```python
from build123d import *

# Parameters (mm, degrees)
F0_R     = 100
F1_DEPTH = 25
F3_DEPTH = 25.5
F4_SIZE  = 5
F5_R     = 5
F6_R     = 30
F7_DEPTH = 25.501


with BuildPart() as f1:
    # F0 (on Front) → F1 (new body)
    with BuildSketch(Plane.XZ):
        Circle(F0_R)
    extrude(amount=F1_DEPTH)

    # F2 (on face) → F3 (join)
    with BuildSketch(Plane.XZ.offset(25)):
        Polygon((-14.1001771265, 119.1687249449), (-19.9524563423, 97.9892825053), (10.5246777377, 99.4446135219), (2.6809251073, 119.9700489313), align=None)
    extrude(amount=-F3_DEPTH)

    # F4
    f4_edges = [f1.edges().sort_by_distance(p)[0] for p in [
        (2.680925, -12.25, 119.970049),
        (-14.100177, -12.25, 119.168725),
    ]]
    chamfer(f4_edges, length=F4_SIZE)

    # F5
    f5_edges = [f1.edges().sort_by_distance(p)[0] for p in [
        (-19.952456, -12.5, 97.989283),
        (10.524678, -12.5, 99.444614),
    ]]
    fillet(f5_edges, radius=F5_R)

    # F6 (on face) + F1_face1 (on face) → F7 (cut, through all)
    with BuildSketch(Plane.XZ.offset(25)):
        Circle(F6_R)
    with BuildSketch(Plane(origin=(0.0031470854, 0, -0.0659053797), x_dir=(1, 0, 0), z_dir=(0, 1, 0))):
        with BuildLine():
            ThreePointArc((13.4432882004, -99.1577485259), (4.7665750707, 99.8202786027), (-22.8304528013, -97.4256204252))
            ThreePointArc((-22.8304528013, -97.4256204252), (-20.5064145734, -98.6893061779), (-19.1524197717, -100.9619155688))
            Line((-19.1524197717, -100.9619155688), (-19.9556034276, -98.055187885))
            Line((-19.9556034276, -98.055187885), (10.5215306523, -99.5105189016))
            Line((10.5215306523, -99.5105189016), (9.4450314489, -102.3274887768))
            ThreePointArc((9.4450314489, -102.3274887768), (11.0094130673, -100.1942364433), (13.4432882004, -99.1577485259))
        make_face()
    extrude(amount=-F7_DEPTH, dir=(0, -1, 0), mode=Mode.SUBTRACT)


solid = f1.part
```
CAD build for the part. Positions are in the model's coordinates, mm. Round coordinates to 2 decimals unless told otherwise and drop trailing zeros. Loops run counter-clockwise (first coordinate to the right, second up) from the corner with the lowest first, then second, coordinate; pieces in that order, holes last. Notation, with made-up numbers: (-0.75, 9.5) - (14.25, 9.5) arc R26 cw to (14.25, 29.5) - close; hole circle Ø4 at (76.5, 56.5). An arc over 180 degrees is marked (long way). Return JSON: item names as keys, results as strings. Group by question number.
Q1. Band-saw the part on D-D on z = 25. Give the cut face in (x, y), plus the area to 3 significant figures.
Q2. Two-plate mould, pull along Z, no slides. Class faces 1 (the face through (-29.97, -12.68, 1.32)), 2 (the face through (6.864, -12.428, 109.023)), 3 (the face through (-5, 0.5, 107)), 4 (the face through (0.6, -12.3, -100)): +Z half, -Z half, draft (parallel to the pull), parting line (faces both ways), or undercut.
Q3. Band-saw the part on C-C on x = 64.5. Give the cut face in (y, z).
Q4. Drill centre lines: line 1 along Y through (x, z) = (-37, 41); line 2 along Z through (x, y) = (0, -8.5); line 3 along X through (y, z) = (-3, 8.5). Where is each one in solid material? Low to high. Write a range as [from, to].
Q5. Flat gauge pins, fed straight in: pin 1 Ø4 at (x, y) = (71, -21.5) entering from -Z; pin 2 Ø10 at (x, y) = (75, -21) entering from -Z; pin 3 Ø10 at (y, z) = (-13, -62.5) entering from -X. Where does each tip first touch, or does it go through?
Q6. Band-saw the part on A-A on z = 0. Give the cut face in (x, y), plus the area to 3 significant figures.
Q7. Band-saw the part on B-B on y = -6.5. Give the cut face in (x, z).
Solutions:
{
 "1": {"outline": "(-96.82, -25) - (-16.58, -25) - (-16.58, 0) - (-96.82, 0) - close; (16.58, -25) - (96.82, -25) - (96.82, 0) - (16.58, 0) - close", "area": "4,010 mm^2"},
 "2": {"face 1": "undercut", "face 2": "+Z half", "face 3": "draft", "face 4": "parting line"},
 "3": {"outline": "(-25, -76.42) - (0, -76.42) - (0, 76.42) - (-25, 76.42) - close"},
 "4": {"line 1": "y = [-25, 0]", "line 2": "z = [-100, -30], [30, 118.22]", "line 3": "x = [-99.64, -28.77], [28.77, 99.64]"},
 "5": {"pin 1": "stops at z = -72.38", "pin 2": "stops at z = -71.41", "pin 3": "stops at x = -81.82"},
 "6": {"outline": "(-100, -25) - (-30, -25) - (-30, 0) - (-100, 0) - close; (30, -25) - (100, -25) - (100, 0) - (30, 0) - close", "area": "3,500 mm^2"},
 "7": {"outline": "(-22.83, 97.36) arc R100 ccw (long way) to (13.45, 99.09) arc R5 cw to (9.45, 102.26) - (4.47, 115.3) - (-2.31, 119.73) - (-9.11, 119.41) - (-15.43, 114.35) - (-19.15, 100.9) arc R5 cw to start; hole circle Ø60 at (0, 0)"}
}
